Can you work these out from the drawing? Everything is in mm from the part's minimum corner. A direction names the side the tool comes from. Give positions to 0.01 mm unless a question says otherwise; leave off trailing zeros. Loops run counter-clockwise (first coordinate to the right, second up) from the corner with the lowest first, then second, coordinate; pieces in that order, holes last.
Q1. If we section it at A-A (y = 26.67): Please give me the cut outline in (x, z), plus the area to 3 significant figures.
Q2. We'd pull the mould along X, two halves only. Please class the marked faces 3, 4 and 5: +X half, -X half, draft (parallel to the pull), parting line (faces both ways), or undercut.
Q3. If we section it at D-D (y = 49.5): Please give me the cut outline in (x, z).
Q4. Will this pin go through, and if not, where does the flat tip stop? P1, Ø12, axis at x = 59, z = 18, coming from the +Y side.
Q5. For the marked faces 1 and 2, which set-ups out of +Z, -Z, +X, -X, +Y, -Y let a thin tool reach every point of the face, with its end or its side?
Q6. I need wall thicknesses on line 1 (X direction, y = 49.5, z = 27.94); line 2 (Y direction, x = 31.5, z = 27.94); line 3 (Z direction, x = 67, y = 26). Which ranges of each line are inside material? Lowest first, please.
Q7. If we section it at B-B (x = 97.5): Please give me the cut outline in (y, z), plus the area to 3 significant figures.
Q8. If we section it at C-C (z = 27.94): Please give me the cut outline in (x, y), plus the area to 3 significant figures.
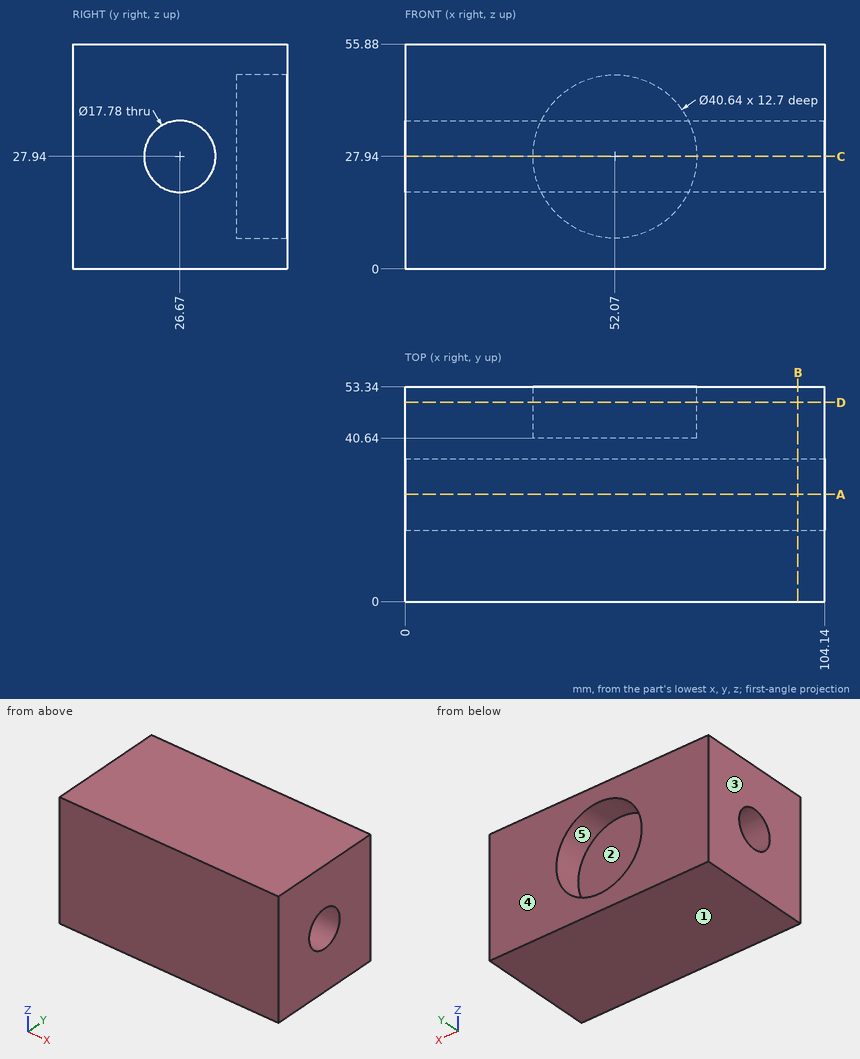
Check sheet entries:
1. outline: (0, 0) - (104.14, 0) - (104.14, 19.05) - (0, 19.05) - close; (0, 36.83) - (104.14, 36.83) - (104.14, 55.88) - (0, 55.88) - close
1. area: 3,970 mm2
2. face 3: -X half
2. face 4: draft
2. face 5: undercut
3. outline: (0, 0) - (104.14, 0) - (104.14, 55.88) - (0, 55.88) - close; hole circle Ø40.64 at (52.07, 27.94)
4. P1: stops at y = 40.64
5. face 1: -Z, +X, -X, +Y, -Y
5. face 2: +Y
6. line 1: x = 0 to 31.75, 72.39 to 104.14
6. line 2: y = 0 to 17.78, 35.56 to 53.34
6. line 3: z = 0 to 19.08, 36.8 to 55.88
7. outline: (0, 0) - (53.34, 0) - (53.34, 55.88) - (0, 55.88) - close; hole circle Ø17.78 at (26.67, 27.94)
7. area: 2,730 mm2
8. outline: (0, 0) - (104.14, 0) - (104.14, 17.78) - (0, 17.78) - close; (0, 35.56) - (104.14, 35.56) - (104.14, 53.34) - (72.39, 53.34) - (72.39, 40.64) - (31.75, 40.64) - (31.75, 53.34) - (0, 53.34) - close
8. area: 3,190 mm2
